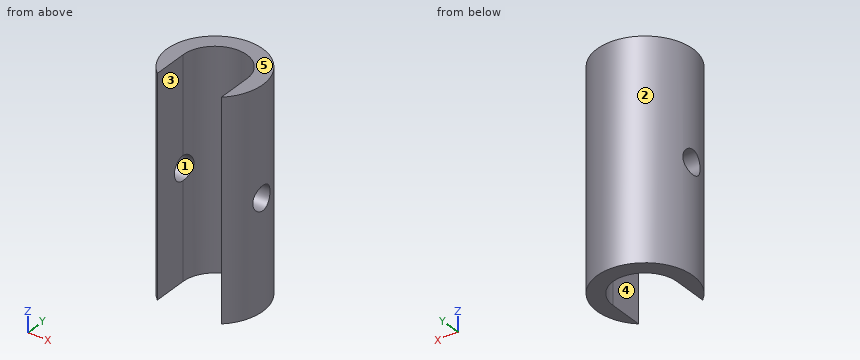
from build123d import *

# Parameters (mm, degrees)
SALIENTE_EXTRUIR1_DEPTH = 27
CROQUIS2_R              = 1.5
CORTAR_EXTRUIR1_DEPTH   = 13.5


with BuildPart() as part:
    # Croquis1 → Saliente-Extruir1 (new body)
    with BuildSketch(Plane(origin=(0, 0, 0), x_dir=(0, 1, 0), z_dir=(0, 0, 1))):
        with BuildLine():
            Line((0, 4), (-4.472135955, 4))
            ThreePointArc((-4.472135955, 4), (6, 0), (-4.472135955, -4))
            Line((-4.472135955, -4), (0, -4))
            ThreePointArc((0, -4), (4, 0), (0, 4))
        make_face()
    extrude(amount=SALIENTE_EXTRUIR1_DEPTH)

    # Croquis2 → Cortar-Extruir1 (cut, symmetric)
    with BuildSketch(Plane.YZ):
        with Locations(Location((0, 13.5, 0), (0, 0, 270))):
            Circle(CROQUIS2_R)
    extrude(amount=CORTAR_EXTRUIR1_DEPTH, both=True, mode=Mode.SUBTRACT)


solid = part.part
Read the model definition and answer for the solid it produces. Units are mm, in the model's axes. Face numbers are marked on the shaded views. A direction names the side the tool comes from. Round coordinates to 2 decimals unless told otherwise and drop trailing zeros. Order: outer loops, then holes, each group sorted by start corner. A loop starts at its lowest first (then second) coordinate and runs counter-clockwise, first axis right, second up. Notation, with made-up numbers: (7.5, 57.5) - (47.5, 57.5) arc R19 cw to (47.5, 80.5) - close; hole circle Ø1 at (88.25, 36). An arc over 180 degrees is marked (long way). Use one line per item in the form item = value. Start each with the question number.
(1) The part is cut by section A-A (z = 13.5). Give the vertices of the cut face in (x, y), then the cut area to 3 significant figures.
(2) The part is cut by section B-B (y = 2.5). Give the vertices of the cut face in (x, z).
(3) The part is cut by section C-C (x = 0). Give the vertices of the cut face in (y, z), then the cut area to 3 significant figures.
(4) The part is cut by section D-D (z = 20). Give the vertices of the cut face in (x, y), then the cut area to 3 significant figures.
(5) For the marked faces 4 and 5, determine the directions among +Z, -Z, +X, -X, +Y, -Y from which every point of the face is accessible in a straight line to the end or side of a thin tool.
(6) Determine the mould class of the marked faces 1, 2 and 3 for opening direction X: +X half, -X half, draft (parallel to the pull), parting line (faces both ways), or undercut.
(7) Flat-ended cylindrical pins translate along their axes: pin 1 Ø2 at (y, z) = (-2, 8.5) entering from -X; pin 2 Ø1.5 at (x, z) = (4, 13) entering from -Y. Find the tip coordinate at first contact, or state that the pin passes through.
(8) Find the intervals of material crossed by line 1 along Z through (x, y) = (-5.5, 0); line 2 along X through (y, z) = (-4, 20.75); line 3 along X through (y, z) = (3.5, 2.75), in increasing order. Write a range as from..to.
Checked values:
q1.outline = (-5.81, -1.5) arc R6 ccw to (-4, -4.47) - (-4, -1.5) - close; (-5.81, 1.5) - (-3.71, 1.5) arc R4 cw to (3.71, 1.5) - (5.81, 1.5) arc R6 ccw to start; (4, -4.47) arc R6 ccw to (5.81, -1.5) - (4, -1.5) - close
q1.area = 31.9 mm^2
q2.outline = (-5.45, 0) - (-3.12, 0) - (-3.12, 27) - (-5.45, 27) - close; (3.12, 0) - (5.45, 0) - (5.45, 27) - (3.12, 27) - close
q3.outline = (4, 0) - (6, 0) - (6, 27) - (4, 27) - close
q3.area = 54.0 mm^2
q4.outline = (-4, -4.47) - (-4, 0) arc R4 cw to (4, 0) - (4, -4.47) arc R6 ccw (long way) to start
q4.area = 43.8 mm^2
q5.face_4 = +Z, -Z, -Y
q5.face_5 = +Z, +X, -X, +Y, -Y
q6.face_1 = draft
q6.face_2 = parting line
q6.face_3 = undercut
q7.pin_1 = -5.92
q7.pin_2 = -4.47
q8.line_1 = 0..12, 15..27
q8.line_2 = -4.47..-4, 4..4.47
q8.line_3 = -4.87..-1.94, 1.94..4.87
